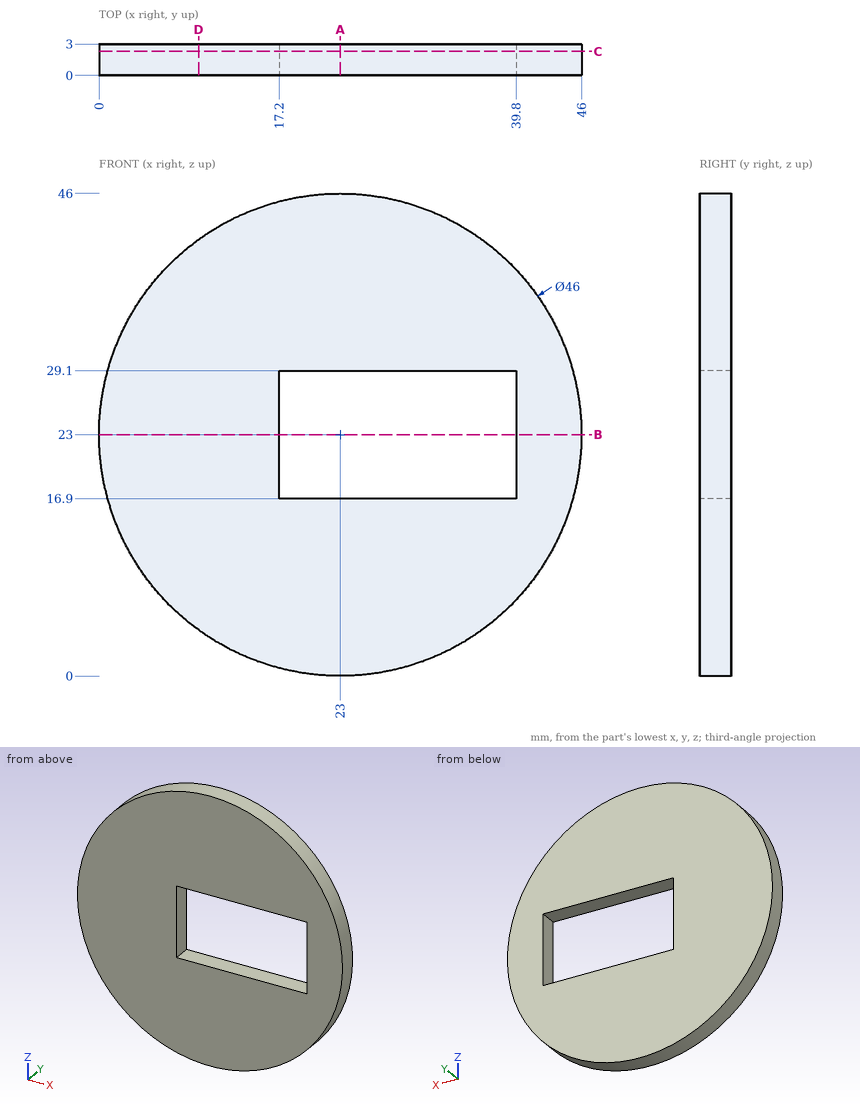
Study the drawing (mm; zero at the part's minimum x, y, z) and answer. Give positions to 0.01 mm unless a question says otherwise; leave off trailing zeros. Loops run counter-clockwise (first coordinate to the right, second up) from the corner with the lowest first, then second, coordinate; pieces in that order, holes last. Notation, with made-up numbers: (79, 40) - (120, 40) arc R31 cw to (120, 67) - close; hole circle Ø9 at (56, 79). An arc over 180 degrees is marked (long way). One line per question, with ' | ' between items.
(1) Straight lines are drawn through the part: probe 1 along Z at (x, y) = (32.5, 1.2); probe 2 along Z at (x, y) = (37.5, 2.4); probe 3 along X at (y, z) = (1.7, 20.5). For each, find the intervals that lie inside material, in ascending order.
Recorded:
probe 1: z = 2.05 to 16.9, 29.1 to 43.95 | probe 2: z = 5.15 to 16.9, 29.1 to 40.85 | probe 3: x = 0.14 to 17.2, 39.8 to 45.86
(2) The part is cut by section B-B (z = 23). Write down the section's boundary in (x, y).
Recorded:
outline: (0, 0) - (17.2, 0) - (17.2, 3) - (0, 3) - close; (39.8, 0) - (46, 0) - (46, 3) - (39.8, 3) - close
(3) The part is cut by section D-D (x = 9.5). Write down the section's boundary in (y, z).
Recorded:
outline: (0, 4.38) - (3, 4.38) - (3, 41.62) - (0, 41.62) - close
(4) Each of these flat-tipped pins is pushed along its axis until it touches: pin 1 Ø0.9 at (x, y) = (27.5, 1) entering from +Z; pin 2 Ø1.5 at (y, z) = (1.5, 6.5) entering from +X. Where does it stop, or does it pass through?
Recorded:
pin 1: stops at z = 45.64 | pin 2: stops at x = 39.76
(5) The part is cut by section A-A (x = 23). Write down the section's boundary in (y, z), then the cut area to 3 significant figures.
Recorded:
outline: (0, 0) - (3, 0) - (3, 16.9) - (0, 16.9) - close; (0, 29.1) - (3, 29.1) - (3, 46) - (0, 46) - close | area: 101 mm²
(6) The part is cut by section C-C (y = 2.3). Write down the section's boundary in (x, z).
Recorded:
outline: circle Ø46 at (23, 23); hole (17.2, 16.9) - (39.8, 16.9) - (39.8, 29.1) - (17.2, 29.1) - close
